Can you work these out from the model? Positions are in its coordinate system, mm. Round coordinates to 2 decimals unless told otherwise and drop trailing zeros. Loops run counter-clockwise (first coordinate to the right, second up) from the corner with the lowest first, then second, coordinate; pieces in that order, holes last. Notation, with made-up numbers: (-34, 18.5) -> (8, 18.5) arc R23 ccw to (8, 42.5) -> close; hole circle Ø5 at (75.5, 10). An arc over 180 degrees is marked (long way). Write item = value, one per line.
from build123d import *

# Parameters (mm, degrees)
F0_W     = 54
F0_H     = 35
F1_DEPTH = 10
F3_D     = 16.5
F5_D     = 6.6


with BuildPart() as f1:
    # F0 (on Top) → F1 (new body)
    with BuildSketch(Plane.XY):
        Rectangle(F0_W, F0_H)
    extrude(amount=F1_DEPTH)

    # F3 (through all)
    with Locations(Plane.XY.offset(10)):
        with Locations((0, 0)):
            Hole(F3_D / 2)

    # F5 (through all)
    with Locations(Plane.XY.offset(10)):
        with Locations((-21, 0), (21, 0)):
            Hole(F5_D / 2)


solid = f1.part
1. We'd pull the mould along Y, two halves only. Please class faces 1 (the flat face through (0, -17.5, 5)), 2 (the cylindrical face through (-7.62, -3.16, 4.93)), 3 (the flat face through (-6, 8, 0)): released by +Y, released by -Y, zero draft, split by the parting line, or undercut.
Entries:
face_1 = released by -Y
face_2 = undercut
face_3 = zero draft
2. Suppose I cut it at B-B, the plane y = 0. List the corners of the cut face in (x, z) for me.
Entries:
outline = (-27, 0) -> (-24.3, 0) -> (-24.3, 10) -> (-27, 10) -> close; (-17.7, 0) -> (-8.25, 0) -> (-8.25, 10) -> (-17.7, 10) -> close; (8.25, 0) -> (17.7, 0) -> (17.7, 10) -> (8.25, 10) -> close; (24.3, 0) -> (27, 0) -> (27, 10) -> (24.3, 10) -> close
3. Suppose I cut it at D-D, the plane y = -5. List the corners of the cut face in (x, z) for me.
Entries:
outline = (-27, 0) -> (-6.56, 0) -> (-6.56, 10) -> (-27, 10) -> close; (6.56, 0) -> (27, 0) -> (27, 10) -> (6.56, 10) -> close
4. I need wall thicknesses on line 1 (Y direction, x = 21, z = 6.5); line 2 (Y direction, x = 0, z = 7); line 3 (X direction, y = 1.5, z = 7). Which ranges of each line are inside material? Lowest first, please. Write a range as [from, to].
Entries:
line_1 = [-17.5, -3.3], [3.3, 17.5]
line_2 = [-17.5, -8.25], [8.25, 17.5]
line_3 = [-27, -23.94], [-18.06, -8.11], [8.11, 18.06], [23.94, 27]
5. Suppose I cut it at C-C, the plane z = 5. List the corners of the cut face in (x, y) for me, and give its area (3 significant figures).
Entries:
outline = (-27, -17.5) -> (27, -17.5) -> (27, 17.5) -> (-27, 17.5) -> close; hole circle Ø6.6 at (-21, 0); hole circle Ø16.5 at (0, 0); hole circle Ø6.6 at (21, 0)
area = 1,610 mm²
6. Suppose I cut it at A-A, the plane x = -21. List the corners of the cut face in (y, z) for me.
Entries:
outline = (-17.5, 0) -> (-3.3, 0) -> (-3.3, 10) -> (-17.5, 10) -> close; (3.3, 0) -> (17.5, 0) -> (17.5, 10) -> (3.3, 10) -> close
